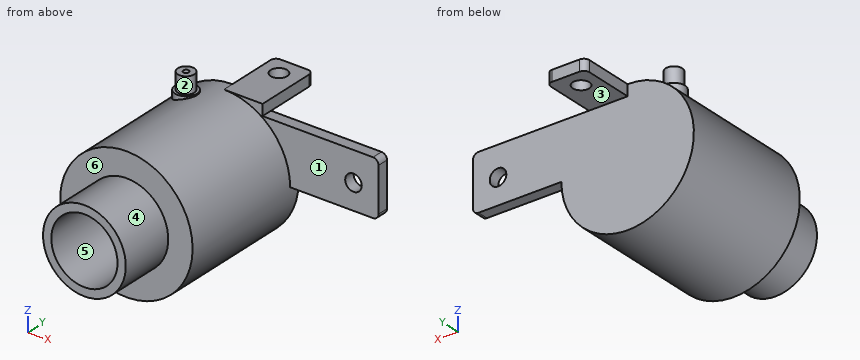
```python
from build123d import *

# Parameters (mm, degrees)
CROQUIS1_W                   = 28
CROQUIS1_H                   = 10
SALIENTE_EXTRUIR1_DEPTH      = 2
CROQUIS5_W                   = 7
CROQUIS5_H                   = 12
SALIENTE_EXTRUIR5_DEPTH      = 2
CROQUIS6_R                   = 12
SALIENTE_EXTRUIR6_DEPTH      = 2
SALIENTE_EXTRUIR6_DEPTH_BACK = 23
CROQUIS9_R                   = 7.5
SALIENTE_EXTRUIR7_DEPTH      = 10
CROQUIS10_R                  = 6
CORTAR_EXTRUIR3_DEPTH        = 33
REDONDEO2_R                  = 1
REDONDEO3_R                  = 1
REDONDEO4_R                  = 1
REDONDEO5_R                  = 1
CROQUIS12_R                  = 1.5
CORTAR_EXTRUIR4_DEPTH        = 2
CROQUIS13_R                  = 1.5
CORTAR_EXTRUIR7_DEPTH        = 2
CROQUIS16_R                  = 2
SALIENTE_EXTRUIR9_DEPTH      = 2
CROQUIS17_R                  = 1.5
SALIENTE_EXTRUIR10_DEPTH     = 5
CROQUIS18_R                  = 0.5
CORTAR_EXTRUIR8_DEPTH        = 5
ESCALA1_SCALE                = 7


with BuildPart() as part:
    # Croquis1 → Saliente-Extruir1 (new body)
    with BuildSketch(Plane(origin=(0, 0, 0), x_dir=(1, 0, 0), z_dir=(0, 1, 0))):
        with Locations((14, 5)):
            Rectangle(CROQUIS1_W, CROQUIS1_H)
    extrude(amount=SALIENTE_EXTRUIR1_DEPTH)

    # Croquis5 → Saliente-Extruir5 (add)
    with BuildSketch(Plane.XY):
        with Locations((3.5, 6)):
            Rectangle(CROQUIS5_W, CROQUIS5_H)
    extrude(amount=SALIENTE_EXTRUIR5_DEPTH)

    # Croquis6 → Saliente-Extruir6 (add, two sides)
    with BuildSketch(Plane(origin=(0, 0, 0), x_dir=(1, 0, 0), z_dir=(0, 1, 0))) as saliente_extruir6_sk:
        with Locations((0, 10)):
            Circle(CROQUIS6_R)
    extrude(amount=SALIENTE_EXTRUIR6_DEPTH)
    extrude(saliente_extruir6_sk.sketch, amount=-SALIENTE_EXTRUIR6_DEPTH_BACK)

    # Croquis9 → Saliente-Extruir7 (add)
    with BuildSketch(Plane(origin=(0, -23, 0), x_dir=(-1, 0, 0), z_dir=(0, -1, 0))):
        with Locations((-0.08521531, 9.936088517)):
            Circle(CROQUIS9_R)
    extrude(amount=SALIENTE_EXTRUIR7_DEPTH)

    # Croquis10 → Cortar-Extruir3 (cut)
    with BuildSketch(Plane.XZ.offset(33)):
        with Locations((0.08521531, -9.936088517)):
            Circle(CROQUIS10_R)
    extrude(amount=-CORTAR_EXTRUIR3_DEPTH, mode=Mode.SUBTRACT)

    # Redondeo2
    redondeo2_edges = [part.edges().sort_by_distance(p)[0] for p in [
        (28, 1, -10),
    ]]
    fillet(redondeo2_edges, radius=REDONDEO2_R)

    # Redondeo3
    redondeo3_edges = [part.edges().sort_by_distance(p)[0] for p in [
        (28, 1, 0),
    ]]
    fillet(redondeo3_edges, radius=REDONDEO3_R)

    # Redondeo4
    redondeo4_edges = [part.edges().sort_by_distance(p)[0] for p in [
        (7, 12, 1),
    ]]
    fillet(redondeo4_edges, radius=REDONDEO4_R)

    # Redondeo5
    redondeo5_edges = [part.edges().sort_by_distance(p)[0] for p in [
        (0, 12, 1),
    ]]
    fillet(redondeo5_edges, radius=REDONDEO5_R)

    # Croquis12 → Cortar-Extruir4 (cut)
    with BuildSketch(Plane.XY):
        with Locations((3.310400977, 8.667805531)):
            Circle(CROQUIS12_R)
    extrude(amount=CORTAR_EXTRUIR4_DEPTH, mode=Mode.SUBTRACT)

    # Croquis13 → Cortar-Extruir7 (cut)
    with BuildSketch(Plane(origin=(0, 0, 0), x_dir=(1, 0, 0), z_dir=(0, 1, 0))):
        with Locations((23.466578788, 5.377069426)):
            Circle(CROQUIS13_R)
    extrude(amount=CORTAR_EXTRUIR7_DEPTH, mode=Mode.SUBTRACT)

    # Croquis16 → Saliente-Extruir9 (add)
    with BuildSketch(Plane.XY):
        with Locations((-4.295016908, -3.333173785)):
            Circle(CROQUIS16_R)
    extrude(amount=SALIENTE_EXTRUIR9_DEPTH)

    # Croquis17 → Saliente-Extruir10 (add)
    with BuildSketch(Plane.XY):
        with Locations((-4.295016908, -3.333173785)):
            Circle(CROQUIS17_R)
    extrude(amount=SALIENTE_EXTRUIR10_DEPTH)

    # Croquis18 → Cortar-Extruir8 (cut)
    with BuildSketch(Plane.XY):
        with Locations((-4.295016908, -3.333173785)):
            Circle(CROQUIS18_R)
    extrude(amount=CORTAR_EXTRUIR8_DEPTH, mode=Mode.SUBTRACT)


with BuildPart() as part_1:
    # Escala1: scaled about (0.668234769, -10.721798359, -9.644957582)
    add(part.part.scale(ESCALA1_SCALE).moved(Location((-4.009408614, 64.330790154, 57.869745492))))


solid = part_1.part
```
For this review, take the finished solid that the model builds, in its own axes (mm). Face numbers are marked on the shaded views. A direction names the side the tool comes from. Round coordinates to 2 decimals unless told otherwise and drop trailing zeros. Write each loop counter-clockwise with the first axis right and the second up, starting at its lowest first coordinate (ties: lowest second). Pieces come first, ordered by that corner, then holes. Notation, with made-up numbers: (77.25, 72) -> (94.25, 72) arc R22 ccw to (94.25, 82) -> close; hole circle Ø8 at (-1, 35.25). An arc over 180 degrees is marked (long way). Use one line per item in the form item = value.
1) Take a section at C-C, the plane x = 105.5. Write out the cut boundary in (y, z), and give its area (3 significant figures).
Found:
outline = (64.33, -12.13) -> (78.33, -12.13) -> (78.33, 57.87) -> (64.33, 57.87) -> close
area = 980 mm2
2) To check wall thickness, follow L1, parallel to Z at x = 16.5, y = 81.5; L2, parallel to X at y = -147.5, z = -49; L3, parallel to Z at x = 129.5, y = 75. State the ranges of each line that lie inside material, in increasing order. Write a range as from..to.
Found:
L1 = 57.87..71.87
L2 = -40.34..-22.69, 15.86..33.52
L3 = -12.13..57.87
3) Take a section at D-D, the plane z = 6. Write out the cut boundary in (x, y), and give its area (3 significant figures).
Found:
outline = (-86.03, -96.67) -> (-52.85, -96.67) -> (-52.85, -166.67) -> (-41.51, -166.67) -> (-41.51, 64.33) -> (34.68, 64.33) -> (34.68, -166.67) -> (46.02, -166.67) -> (46.02, -96.67) -> (78.01, -96.67) -> (78.01, 64.33) -> (191.99, 64.33) -> (191.99, 78.33) -> (-86.03, 78.33) -> close
area = 19,600 mm2
4) Clearance check with flat-ended pins moving along their axes: pin 1 (2 mm diameter, centred on x = 9.5, z = 35.5, fed in from +Y); pin 2 (15.5 mm diameter, centred on x = 125, y = 72.5, fed in from +Z); pin 3 (25 mm diameter, centred on x = 47, z = 29.5, fed in from -Y); pin 4 (12.5 mm diameter, centred on x = 160.26, z = 20.23, fed in from +Y). State where each tip first meets the part, or that it passes through.
Found:
pin_1 = 78.33
pin_2 = 57.87
pin_3 = -96.67
pin_4 = through
5) Take a section at B-B, the plane y = 104. Write out the cut boundary in (x, z).
Found:
outline = (-4.01, 57.87) -> (44.99, 57.87) -> (44.99, 71.87) -> (-4.01, 71.87) -> close
6) Tool access review of the marked faces 1, 2 and 3: name each direction out of +Z, -Z, +X, -X, +Y, -Y from which nothing blocks a thin tool from reaching the whole face with its end or side.
Found:
face_1 = +Z, +X, -Y
face_2 = +Z
face_3 = -Z, +X, -X, +Y
7) Mouldability with a two-part tool opening along X and no side actions: class the marked faces 4, 5 and 6 as +X half, -X half, draft (parallel to the pull), parting line (faces both ways), or undercut.
Found:
face_4 = parting line
face_5 = undercut
face_6 = draft
8) Take a section at A-A, the plane x = 157. Write out the cut boundary in (y, z), and give its area (4 significant figures).
Found:
outline = (64.33, -12.13) -> (78.33, -12.13) -> (78.33, 10.25) -> (64.33, 10.25) -> close; (64.33, 30.21) -> (78.33, 30.21) -> (78.33, 57.87) -> (64.33, 57.87) -> close
area = 700.5 mm2
